Part model, mm, in its own coordinate system. A direction names the side the tool comes from. Give positions to 0.01 mm unless a question says otherwise; leave off trailing zeros. Order: outer loops, then holes, each group sorted by start corner. A loop starts at its lowest first (then second) coordinate and runs counter-clockwise, first axis right, second up. Notation, with made-up numbers: (59.5, 40) - (86.5, 40) arc R31 cw to (86.5, 76) - close; hole circle Ø8 at (38.25, 74). An arc over 180 degrees is marked (long way). Use one line per item in the form item = value. Start each with the question number.
1. Band-saw the part on D-D, the plane y = -58.5. List the corners of the cut face in (x, z).
2. Tool access for faces 4 (the face through (-29.76, 12.52, 35.48)), 5 (the face through (-44.112, -63, 23)), 6 (the face through (-31.412, -26, 23)): list every direction of +Z, -Z, +X, -X, +Y, -Y with a clear straight run to the whole face (end or side of a thin tool).
3. Pin check, flat tips, straight feed: P1, Ø8, axis at x = -17, z = 3, coming from the +Y side; P2, Ø7.5, axis at x = -29, y = -61, coming from the +Z side; P3, Ø12.5, axis at x = -28, y = -63, coming from the -Z side. Stop position of each tip, or through.
4. Band-saw the part on B-B, the plane x = -29. List the corners of the cut face in (y, z), plus the area to 3 significant figures.
5. Drill centre lines: line 1 (Z direction, x = -12.5, y = -25.4); line 2 (Y direction, x = -54, z = 37.5); line 3 (X direction, y = -25, z = 22.5). Where is each one in solid material? Low to high.
6. Pull direction Z, two halves, no side cores. Call faces 1 (the face through (-32, -63, 35.586)), 2 (the face through (-18.534, -18.573, 33.595)), 3 (the face through (-18.712, -63, 23)): +Z half, -Z half, draft (parallel to the pull), parting line (faces both ways), or undercut.
7. Band-saw the part on C-C, the plane z = 20. List the corners of the cut face in (x, y), plus the area to 3 significant figures.
8. Band-saw the part on A-A, the plane y = -25.4. List the corners of the cut face in (x, z), plus the area to 3 significant figures.
from build123d import *

# Parameters (mm, degrees)
F0_W     = 50.8
F0_H     = 50.8
F1_DEPTH = 50.8
F2_W     = 25.4
F2_H     = 25.4
F3_DEPTH = 25.4
F4_R     = 12.7
F5_DEPTH = 25.4
F6_R     = 12.7
F7_DEPTH = 25.4


with BuildPart() as f1:
    # F0 (on Front) → F1 (new body)
    with BuildSketch(Plane.XZ):
        with Locations((-31.411681, 22.886025)):
            Rectangle(F0_W, F0_H)
    extrude(amount=F1_DEPTH)

    # F2 (on face) → F3 (join)
    with BuildSketch(Plane.XZ.offset(50.8)):
        with Locations((-31.411681, 22.886025)):
            Rectangle(F2_W, F2_H)
    extrude(amount=F3_DEPTH)

    # F4 (on face) → F5 (cut)
    with BuildSketch(Plane.YZ.offset(-6.011681)):
        with Locations((-25.4, 22.886025)):
            Circle(F4_R)
    extrude(amount=-F5_DEPTH, mode=Mode.SUBTRACT)

    # F6 (on face) → F7 (join)
    with BuildSketch(Plane(origin=(0, 0, 0), x_dir=(-1, 0, 0), z_dir=(0, 1, 0))):
        with Locations((31.411681, 22.886025)):
            Circle(F6_R)
    extrude(amount=F7_DEPTH)


solid = f1.part
From the geometry:
q1.outline = (-44.11, 10.19) - (-18.71, 10.19) - (-18.71, 35.59) - (-44.11, 35.59) - close
q2.face_4 = +Y
q2.face_5 = +Z, -Z, -X, -Y
q2.face_6 = +X
q3.P1 = 0
q3.P2 = 35.59
q3.P3 = 10.19
q4.outline = (-76.2, 10.19) - (-50.8, 10.19) - (-50.8, -2.51) - (0, -2.51) - (0, 10.42) - (25.4, 10.42) - (25.4, 35.35) - (0, 35.35) - (0, 48.29) - (-50.8, 48.29) - (-50.8, 35.59) - (-76.2, 35.59) - close; hole circle Ø25.4 at (-25.4, 22.89)
q4.area = 3,350 mm²
q5.line_1 = -2.51 to 10.19, 35.59 to 48.29
q5.line_2 = -50.8 to 0
q5.line_3 = -56.81 to -31.41
q6.face_1 = +Z half
q6.face_2 = undercut
q6.face_3 = draft
q7.outline = (-56.81, -50.8) - (-44.11, -50.8) - (-44.11, -76.2) - (-18.71, -76.2) - (-18.71, -50.8) - (-6.01, -50.8) - (-6.01, -37.77) - (-31.41, -37.77) - (-31.41, -13.03) - (-6.01, -13.03) - (-6.01, 0) - (-19.04, 0) - (-19.04, 25.4) - (-43.78, 25.4) - (-43.78, 0) - (-56.81, 0) - close
q7.area = 3,230 mm²
q8.outline = (-56.81, -2.51) - (-6.01, -2.51) - (-6.01, 10.19) - (-31.41, 10.19) - (-31.41, 35.59) - (-6.01, 35.59) - (-6.01, 48.29) - (-56.81, 48.29) - close
q8.area = 1,940 mm²
